The drawing under review shows one solid part. Ordinate dimensions are in mm from its lowest x, y, z. A direction names the side the tool comes from. Round coordinates to 2 decimals unless told otherwise and drop trailing zeros. Order: outer loops, then holes, each group sorted by start corner. A loop starts at its lowest first (then second) coordinate and runs counter-clockwise, first axis right, second up. Notation, with made-up numbers: M 85.5,41 L 139.5,41 A31 ccw 139.5,70 Z; hole C 6.25,40.5 d6. An arc over 180 degrees is marked long. Answer as a JSON object with one key per item and string values. Group by question number.
1) Consider section C-C, the plane x = 22.25. Write out the cut boundary in (y, z), then the cut area to 3 significant figures.
2) For the marked faces 4, 5 and 6, list the 3-axis set-ups (+Z, -Z, +X, -X, +Y, -Y) from which the entire face can be reached by the end or side of a thin tool; tool diameter is ignored.
3) The part is to be moulded in two halves that separate along X. For the marked faces 1, 2 and 3, say which applies: +X half, -X half, draft (parallel to the pull), parting line (faces both ways), or undercut.
4) Consider section B-B, the plane z = 1. Write out the cut boundary in (x, y).
5) Insertion check: pin 1 Ø3 at (x, y) = (22, 4.5) entering from -Z; pin 2 Ø1.8 at (x, z) = (1, 3) entering from -Y; pin 3 Ø5 at (x, z) = (16, 3) entering from -Y. Each pin has a flat end and moves straight along its axis. Give the tip position at first contact, or say it passes through.
6) Consider section D-D, the plane y = 8.25. Write out the cut boundary in (x, z), then the cut area to 3 significant figures.
7) Consider section A-A, the plane x = 13.5. Write out the cut boundary in (y, z).
8) To check wall thickness, follow line 1 (Y direction, x = 13.5, z = 9); line 2 (Y direction, x = 12.75, z = 3.5); line 3 (Y direction, x = 8.25, z = 9.25). State the ranges of each line that lie inside material, in increasing order.
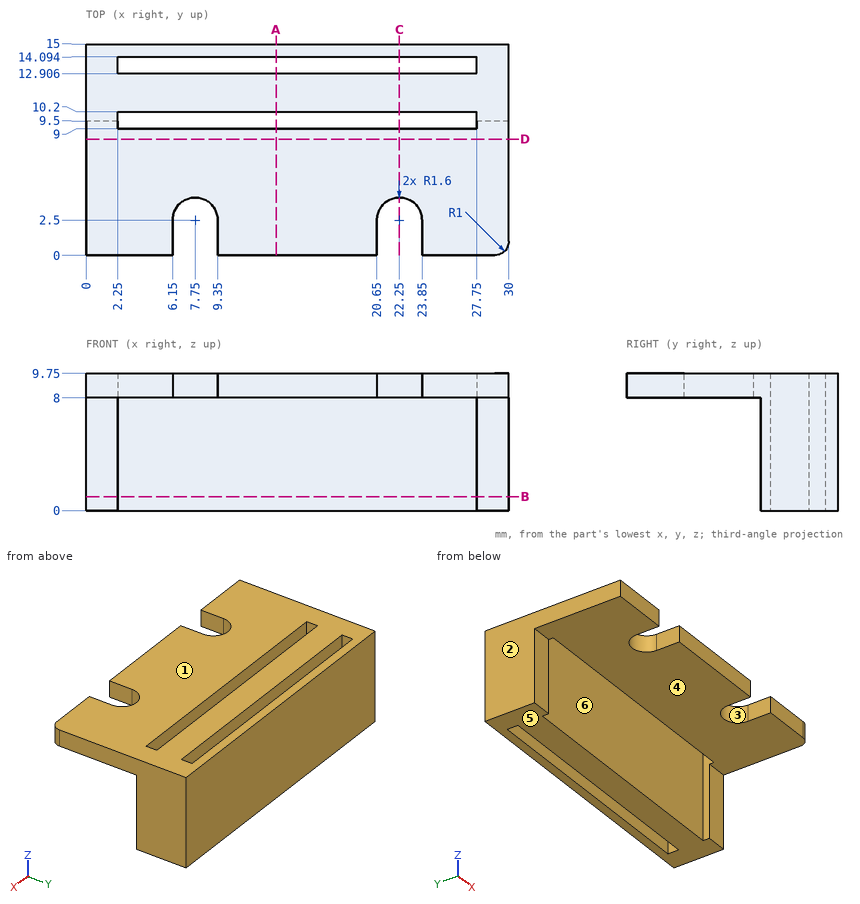
Results list:
{
 "1": {"outline": "M 4.1,8 L 9,8 L 9,9.75 L 4.1,9.75 Z; M 10.2,0 L 12.91,0 L 12.91,9.75 L 10.2,9.75 Z; M 14.09,0 L 15,0 L 15,9.75 L 14.09,9.75 Z", "area": "43.8 mm^2"},
 "2": {"face 4": "-Z, +X, -X, -Y", "face 5": "-Z, +X, -X, +Y, -Y", "face 6": "+Z, -Z"},
 "3": {"face 1": "draft", "face 2": "-X half", "face 3": "undercut"},
 "4": {"outline": "M 0,9.5 L 2.25,9.5 L 2.25,10.2 L 27.75,10.2 L 27.75,9.5 L 30,9.5 L 30,15 L 0,15 Z; hole M 2.25,12.91 L 27.75,12.91 L 27.75,14.09 L 2.25,14.09 Z"},
 "5": {"pin 1": "z = 8", "pin 2": "y = 9.5", "pin 3": "y = 10.2"},
 "6": {"outline": "M 0,8 L 30,8 L 30,9.75 L 0,9.75 Z", "area": "52.5 mm^2"},
 "7": {"outline": "M 0,8 L 9,8 L 9,9.75 L 0,9.75 Z; M 10.2,0 L 12.91,0 L 12.91,9.75 L 10.2,9.75 Z; M 14.09,0 L 15,0 L 15,9.75 L 14.09,9.75 Z"},
 "8": {"line 1": "0 to 9, 10.2 to 12.91, 14.09 to 15", "line 2": "10.2 to 12.91, 14.09 to 15", "line 3": "4.02 to 9, 10.2 to 12.91, 14.09 to 15"}
}
